The figure shows three views and two pictorial views of one solid part (mm, origin at its lowest corner). Answer the questions. A direction names the side the tool comes from. Give positions to 0.01 mm unless a question says otherwise; leave off trailing zeros. Loops run counter-clockwise (first coordinate to the right, second up) from the corner with the lowest first, then second, coordinate; pieces in that order, holes last. Notation, with made-up numbers: (-3, 34.5) - (33, 34.5) arc R15 ccw to (33, 52.5) - close; hole circle Ø2 at (12, 34.5). An arc over 180 degrees is marked (long way). Write each question's results on one line, items separated by ' | '.
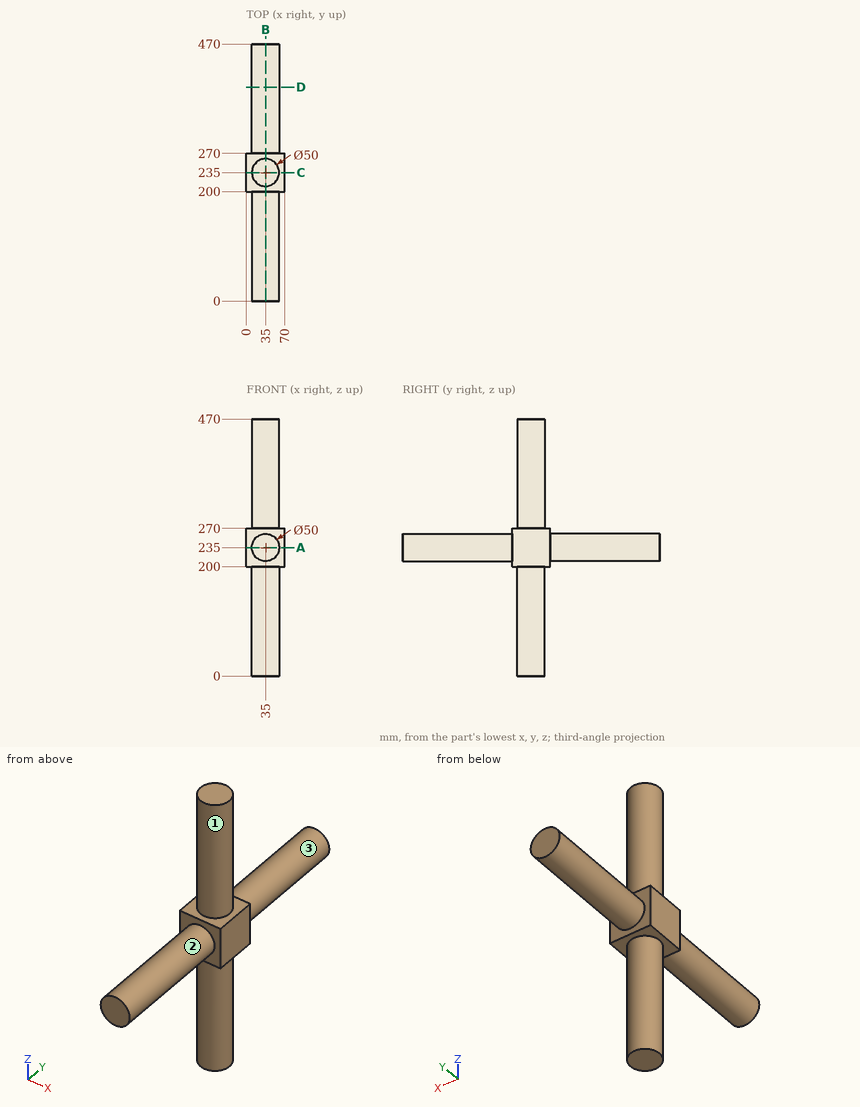
Item 1: Find the intervals of material crossed by line 1 along Y through (x, z) = (36, 169); line 2 along Y through (x, z) = (21.5, 126); line 3 along Z through (x, y) = (46.5, 52), in increasing order. Write a range as [from, to].
Values found:
line 1: y = [210.02, 259.98] | line 2: y = [213.96, 256.04] | line 3: z = [212.8, 257.2]
Item 2: A cutting plane is placed at D-D, the plane y = 391. Determine the outline of the cut face in (x, z), plus the area to 3 significant figures.
Values found:
outline: circle Ø50 at (35, 235) | area: 1,960 mm²
Item 3: For the marked faces 1, 2 and 3, determine the directions among +Z, -Z, +X, -X, +Y, -Y from which every point of the face is accessible in a straight line to the end or side of a thin tool.
Values found:
face 1: +Z | face 2: -Y | face 3: +Y
Item 4: Flat-ended cylindrical pins translate along their axes: P1, Ø2, axis at x = 17, y = 355, coming from the +Z side; P2, Ø1, axis at x = 25.5, y = 113, coming from the -Z side; P3, Ø4, axis at x = 62.5, z = 119, coming from the -Y side; P4, Ø2, axis at x = 46.5, y = 110.5, coming from the -Z side. Find the tip coordinate at first contact, or state that the pin passes through.
Values found:
P1: stops at z = 253.33 | P2: stops at z = 211.68 | P3: passes through | P4: stops at z = 212.31
Item 5: A cutting plane is placed at B-B, the plane x = 35. Determine the outline of the cut face in (y, z), plus the area to 3 significant figures.
Values found:
outline: (0, 210) - (200, 210) - (200, 200) - (210, 200) - (210, 0) - (260, 0) - (260, 200) - (270, 200) - (270, 210) - (470, 210) - (470, 260) - (270, 260) - (270, 270) - (260, 270) - (260, 470) - (210, 470) - (210, 270) - (200, 270) - (200, 260) - (0, 260) - close | area: 44,900 mm²
Item 6: A cutting plane is placed at A-A, the plane z = 235. Determine the outline of the cut face in (x, y).
Values found:
outline: (0, 200) - (10, 200) - (10, 0) - (60, 0) - (60, 200) - (70, 200) - (70, 270) - (60, 270) - (60, 470) - (10, 470) - (10, 270) - (0, 270) - close
